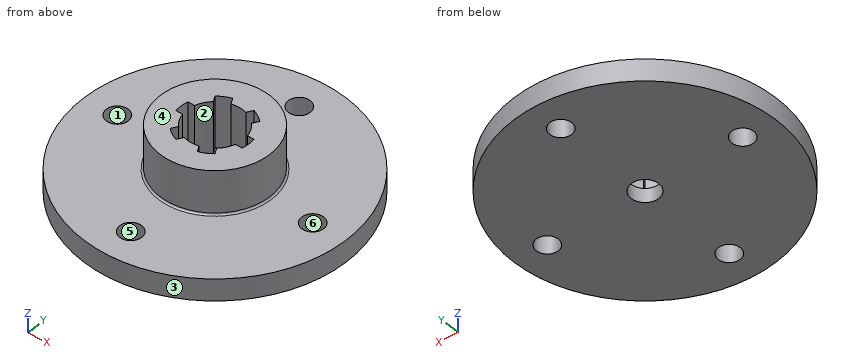
from build123d import *

# Parameters (mm, degrees)
SKETCH1_W           = 38.1
SKETCH1_H           = 6.35
SKETCH2_R           = 15.875
BOSS_EXTRUDE1_DEPTH = 12.7
CUT_EXTRUDE1_DEPTH  = 14.986
HOLE1_D             = 6.35
SKETCH10_R          = 4
CUT_EXTRUDE3_DEPTH  = 10
FILLET2_R           = 0.5


with BuildPart() as part:
    # Sketch1 → Revolve1 (revolve)
    with BuildSketch(Plane(origin=(0, 0, 0), x_dir=(1, 0, 0), z_dir=(0, 1, 0))):
        with Locations((19.05, 0)):
            Rectangle(SKETCH1_W, SKETCH1_H)
    revolve(axis=Axis((0, 0, -3.175), (0, 0, 1)))

    # Sketch2 → Boss-Extrude1 (add)
    with BuildSketch(Plane.XY.offset(3.175)):
        Circle(SKETCH2_R)
    extrude(amount=BOSS_EXTRUDE1_DEPTH)

    # Sketch3 → Cut-Extrude1 (cut)
    with BuildSketch(Plane.XY.offset(15.875)):
        with BuildLine():
            Line((-7.813605563, 2.134846154), (-9.769464259, 2.134846154))
            ThreePointArc((-9.769464259, 2.134846154), (-9.999052891, 0.137627323), (-9.824520402, -1.865153846))
            Line((-9.824520402, -1.865153846), (-7.882334751, -1.865153846))
            ThreePointArc((-7.882334751, -1.865153846), (-7.083348537, -3.928889601), (-5.755633784, -5.699357836))
            Line((-5.755633784, -5.699357836), (-6.733563132, -7.393181152))
            ThreePointArc((-6.733563132, -7.393181152), (-5.118715203, -8.590620156), (-3.296989588, -9.440861171))
            Line((-3.296989588, -9.440861171), (-2.325896763, -7.758879059))
            ThreePointArc((-2.325896763, -7.758879059), (-0.139156065, -8.098804578), (2.057971779, -7.83420399))
            Line((2.057971779, -7.83420399), (3.035901127, -9.528027306))
            ThreePointArc((3.035901127, -9.528027306), (4.880337688, -8.728247479), (6.527530814, -7.575707325))
            Line((6.527530814, -7.575707325), (5.556437988, -5.893725213))
            ThreePointArc((5.556437988, -5.893725213), (6.944192472, -4.169914977), (7.813605563, -2.134846154))
            Line((7.813605563, -2.134846154), (9.769464259, -2.134846154))
            ThreePointArc((9.769464259, -2.134846154), (9.999052891, -0.137627323), (9.824520402, 1.865153846))
            Line((9.824520402, 1.865153846), (7.882334751, 1.865153846))
            ThreePointArc((7.882334751, 1.865153846), (7.083348537, 3.928889601), (5.755633784, 5.699357836))
            Line((5.755633784, 5.699357836), (6.733563132, 7.393181152))
            ThreePointArc((6.733563132, 7.393181152), (5.118715203, 8.590620156), (3.296989588, 9.440861171))
            Line((3.296989588, 9.440861171), (2.325896763, 7.758879059))
            ThreePointArc((2.325896763, 7.758879059), (0.139156065, 8.098804578), (-2.057971779, 7.83420399))
            Line((-2.057971779, 7.83420399), (-3.035901127, 9.528027306))
            ThreePointArc((-3.035901127, 9.528027306), (-4.880337688, 8.728247479), (-6.527530814, 7.575707325))
            Line((-6.527530814, 7.575707325), (-5.556437988, 5.893725213))
            ThreePointArc((-5.556437988, 5.893725213), (-6.944192472, 4.169914977), (-7.813605563, 2.134846154))
        make_face()
    extrude(amount=-CUT_EXTRUDE1_DEPTH, mode=Mode.SUBTRACT)

    # Hole1 (through all)
    with Locations(Plane(origin=(0, 0, -3.175), x_dir=(-1, 0, 0), z_dir=(0, 0, -1))):
        with Locations((0, 28.575), (-28.575, 0), (28.575, 0), (0, -28.575)):
            Hole(HOLE1_D / 2)

    # Sketch10 → Cut-Extrude3 (cut)
    with BuildSketch(Plane.XY.offset(0.889)):
        Circle(SKETCH10_R)
    extrude(amount=-CUT_EXTRUDE3_DEPTH, mode=Mode.SUBTRACT)

    # Fillet2
    fillet2_edges = [part.edges().sort_by_distance(p)[0] for p in [
        (-15.875, 0, 3.175),
    ]]
    fillet(fillet2_edges, radius=FILLET2_R)


solid = part.part
Could you check a few things on this model? Use its own coordinates, in mm. Face numbers are marked on the shaded views. A direction names the side the tool comes from. Give positions to 0.01 mm unless a question says otherwise; leave off trailing zeros. Order: outer loops, then holes, each group sorted by start corner. A loop starts at its lowest first (then second) coordinate and runs counter-clockwise, first axis right, second up.
1. For pin 1 (10 mm diameter, centred on x = -28.575, y = 0, fed in from +Z) (3 decimals); pin 2 (10 mm diameter, centred on x = 0, y = 28.575, fed in from -Z) (3 decimals); pin 3 (3 mm diameter, centred on y = 3, z = 8.5, fed in from +X); pin 4 (0.6 mm diameter, centred on x = -9, z = 12, fed in from +Y), each with a flat end and sliding along its axis, tell me the tip position at first contact or that it passes through.
Answers below:
pin 1: stops at z = 3.175
pin 2: stops at z = -3.175
pin 3: stops at x = 15.8
pin 4: stops at y = 13.28
2. Suppose I cut it at D-D (z = -0.5). Write out the boundary of the cut face in (x, y) (3 decimals), plus the area to 3 significant figures.
Answers below:
outline: circle Ø76.2 at (0, 0); hole circle Ø6.35 at (-28.575, 0); hole circle Ø8 at (0, 0); hole circle Ø6.35 at (0, -28.575); hole circle Ø6.35 at (0, 28.575); hole circle Ø6.35 at (28.575, 0)
area: 4,380 mm2
3. Suppose I cut it at A-A (x = 0). Write out the boundary of the cut face in (y, z) (3 decimals).
Answers below:
outline: (-38.1, -3.175) - (-31.75, -3.175) - (-31.75, 3.175) - (-38.1, 3.175) - close; (-25.4, -3.175) - (-4, -3.175) - (-4, 0.889) - (-8.1, 0.889) - (-8.1, 15.875) - (-15.875, 15.875) - (-15.875, 3.675) arc R0.5 cw to (-16.375, 3.175) - (-25.4, 3.175) - close; (4, -3.175) - (25.4, -3.175) - (25.4, 3.175) - (16.375, 3.175) arc R0.5 cw to (15.875, 3.675) - (15.875, 15.875) - (8.1, 15.875) - (8.1, 0.889) - (4, 0.889) - close; (31.75, -3.175) - (38.1, -3.175) - (38.1, 3.175) - (31.75, 3.175) - close
4. Suppose I cut it at B-B (y = 0). Write out the boundary of the cut face in (x, z) (3 decimals), plus the area to 3 significant figures.
Answers below:
outline: (-38.1, -3.175) - (-31.75, -3.175) - (-31.75, 3.175) - (-38.1, 3.175) - close; (-25.4, -3.175) - (-4, -3.175) - (-4, 0.889) - (-10, 0.889) - (-10, 15.875) - (-15.875, 15.875) - (-15.875, 3.675) arc R0.5 cw to (-16.375, 3.175) - (-25.4, 3.175) - close; (4, -3.175) - (25.4, -3.175) - (25.4, 3.175) - (16.375, 3.175) arc R0.5 cw to (15.875, 3.675) - (15.875, 15.875) - (10, 15.875) - (10, 0.889) - (4, 0.889) - close; (31.75, -3.175) - (38.1, -3.175) - (38.1, 3.175) - (31.75, 3.175) - close
area: 474 mm2
5. Which directions (+Z, -Z, +X, -X, +Y, -Y) give clear straight access to the entire face, cutting with the end or side of a thin tool? Please do the marked faces 1 and 2.
Answers below:
face 1: +Z, -Z
face 2: +Z
6. I need wall thicknesses on L1, parallel to Y at x = 0, z = 1.5; L2, parallel to Y at x = -2.5, z = 1.25; L3, parallel to X at y = -2.5, z = 1. Which ranges of each line are inside material? Lowest first, please.
Answers below:
L1: y = -38.1 to -31.75, -25.4 to -8.1, 8.1 to 25.4, 31.75 to 38.1
L2: y = -38.02 to -30.53, -26.62 to -8.06, 8.6 to 26.62, 30.53 to 38.02
L3: x = -38.02 to -30.53, -26.62 to -7.7, 7.7 to 26.62, 30.53 to 38.02
7. Thinking about a two-plate mould opening in X: for the marked faces 3, 4, 5 and 6, which applies, +X half, -X half, draft (parallel to the pull), parting line (faces both ways), or undercut?
Answers below:
face 3: parting line
face 4: draft
face 5: undercut
face 6: undercut
8. Suppose I cut it at C-C (z = 14.5). Write out the boundary of the cut face in (x, y) (3 decimals).
Answers below:
outline: circle Ø31.75 at (0, 0); hole (-9.825, -1.865) - (-7.882, -1.865) arc R8.1 ccw to (-5.756, -5.699) - (-6.734, -7.393) arc R10 ccw to (-3.297, -9.441) - (-2.326, -7.759) arc R8.1 ccw to (2.058, -7.834) - (3.036, -9.528) arc R10 ccw to (6.528, -7.576) - (5.556, -5.894) arc R8.1 ccw to (7.814, -2.135) - (9.769, -2.135) arc R10 ccw to (9.825, 1.865) - (7.882, 1.865) arc R8.1 ccw to (5.756, 5.699) - (6.734, 7.393) arc R10 ccw to (3.297, 9.441) - (2.326, 7.759) arc R8.1 ccw to (-2.058, 7.834) - (-3.036, 9.528) arc R10 ccw to (-6.528, 7.576) - (-5.556, 5.894) arc R8.1 ccw to (-7.814, 2.135) - (-9.769, 2.135) arc R10 ccw to start
